from build123d import *

# Parameters (mm, degrees)
SKETCH1_W           = 52
SKETCH1_H           = 50
BOSS_EXTRUDE1_DEPTH = 5
SKETCH2_W           = 52
SKETCH2_H           = 15
BOSS_EXTRUDE2_DEPTH = 131
CUT_EXTRUDE1_DEPTH  = 50
SKETCH4_W           = 10
SKETCH4_H           = 2
CUT_EXTRUDE2_DEPTH  = 81


with BuildPart() as part:
    # Sketch1 → Boss-Extrude1 (new body)
    with BuildSketch(Plane(origin=(0, 0, 0), x_dir=(1, 0, 0), z_dir=(0, 1, 0))):
        Rectangle(SKETCH1_W, SKETCH1_H)
    extrude(amount=BOSS_EXTRUDE1_DEPTH)

    # Sketch2 → Boss-Extrude2 (add)
    with BuildSketch(Plane(origin=(0, 5, 0), x_dir=(1, 0, 0), z_dir=(0, 1, 0))):
        with Locations((0, 17.5)):
            Rectangle(SKETCH2_W, SKETCH2_H)
    extrude(amount=BOSS_EXTRUDE2_DEPTH)

    # Sketch3 → Cut-Extrude1 (cut)
    with BuildSketch(Plane(origin=(0, 136, 0), x_dir=(1, 0, 0), z_dir=(0, 1, 0))):
        Polygon((-5, 10), (5, 10), (5, 15), (9, 15), (5, 20), (-5, 20), (-9, 15), (-5, 15), align=None)
    extrude(amount=-CUT_EXTRUDE1_DEPTH, mode=Mode.SUBTRACT)

    # Sketch4 → Cut-Extrude2 (cut)
    with BuildSketch(Plane(origin=(0, 86, 0), x_dir=(1, 0, 0), z_dir=(0, 1, 0))):
        with Locations((0, 11)):
            Rectangle(SKETCH4_W, SKETCH4_H)
    extrude(amount=-CUT_EXTRUDE2_DEPTH, mode=Mode.SUBTRACT)


solid = part.part
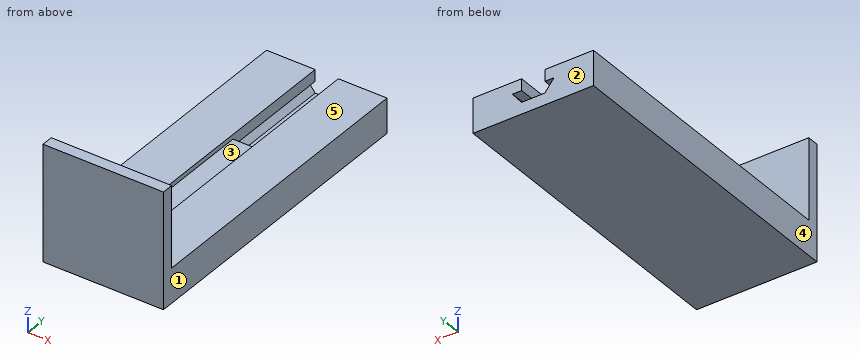
Verification items for the finished model (mm, model axes). Face numbers are marked on the shaded views. A direction names the side the tool comes from. Coordinates: 2 decimals unless noted, no trailing zeros. Order: outer loops, then holes, each group sorted by start corner. A loop starts at its lowest first (then second) coordinate and runs counter-clockwise, first axis right, second up.
1. Go/stop test with flat-tipped pins: pin 1 Ø8 at (x, y) = (-1.5, 53.5) entering from +Z; pin 2 Ø1 at (x, z) = (-1, -9) entering from +Y; pin 3 Ø3 at (x, z) = (-14.5, 19.5) entering from -Y; pin 4 Ø2.5 at (x, z) = (2, -14) entering from +Y. Record where each tip stops, or that it passes through.
Results found:
pin 1: stops at z = -10
pin 2: stops at y = 5
pin 3: stops at y = 0
pin 4: stops at y = 86
2. Sectioned sample at A-A, the plane y = 61. Record the cut outline in (x, z).
Results found:
outline: (-26, -25) - (26, -25) - (26, -10) - (5, -10) - (5, -12) - (-5, -12) - (-5, -10) - (-26, -10) - close
3. Sectioned sample at C-C, the plane z = 9. Record the cut outline in (x, y), and give its area (3 significant figures).
Results found:
outline: (-26, 0) - (26, 0) - (26, 5) - (-26, 5) - close
area: 260 mm2
4. Scan lines: line 1 (X direction, y = 38, z = -11); line 2 (Y direction, x = -22.5, z = 17); line 3 (Z direction, x = 8, y = 71.5). Record each from-to range of solid material in increasing order.
Results found:
line 1: x = -26 to -5, 5 to 26
line 2: y = 0 to 5
line 3: z = -25 to -10
5. Sectioned sample at B-B, the plane x = 17.5. Record the cut outline in (y, z), and give its area (4 significant figures).
Results found:
outline: (0, -25) - (136, -25) - (136, -10) - (5, -10) - (5, 25) - (0, 25) - close
area: 2,215 mm2
6. Sectioned sample at D-D, the plane y = 113. Record the cut outline in (x, z), and give its area (3 significant figures).
Results found:
outline: (-26, -25) - (26, -25) - (26, -10) - (5, -10) - (5, -15) - (9, -15) - (5, -20) - (-5, -20) - (-9, -15) - (-5, -15) - (-5, -10) - (-26, -10) - close
area: 660 mm2
7. Release check for a two-part mould opening along X. For the marked faces 1, 2 and 3 record: +X half, -X half, draft (parallel to the pull), parting line (faces both ways), or undercut.
Results found:
face 1: +X half
face 2: draft
face 3: undercut
8. Set-up check for the marked faces 4 and 5: record each of +Z, -Z, +X, -X, +Y, -Y from which the full face is reachable in a straight line by a thin tool's end or side.
Results found:
face 4: +Z, -Z, -X, +Y, -Y
face 5: +Z, +X, -X, +Y
